Read the model definition and answer for the solid it produces. Units are mm, in the model's axes. A direction names the side the tool comes from. Give positions to 0.01 mm unless a question says otherwise; leave off trailing zeros. Order: outer loops, then holes, each group sorted by start corner. A loop starts at its lowest first (then second) coordinate and runs counter-clockwise, first axis right, second up. Notation, with made-up numbers: M 14,13.25 L 24,13.25 A19 ccw 24,19.25 Z; hole C 20,45.5 d5. An arc over 180 degrees is marked long. Write item = value, one per line. Start each with the question number.
from build123d import *

# Parameters (mm, degrees)
F1_DEPTH = 12.7


with BuildPart() as f1:
    # F0 (on Front) → F1 (new body)
    with BuildSketch(Plane.XZ):
        Polygon((44.074243, -1.927952), (-13.075757, -1.927952), (-13.075757, -8.277952), (15.499243, -8.277952), (44.074243, -8.277952), align=None)
        Polygon((15.499243, -8.277952), (-13.075757, -8.277952), (-41.650757, -8.277952), (-41.650757, -14.627952), (15.499243, -14.627952), align=None)
        Polygon((72.649243, -8.277952), (44.074243, -8.277952), (15.499243, -8.277952), (15.499243, -14.627952), (72.649243, -14.627952), align=None)
    extrude(amount=F1_DEPTH)


solid = f1.part
1) Find section C-C on x = -24. Determine the outline of the cut face in (y, z).
2) For a pull along Y with two mould halves and no side action, classify faces 1 (the face through (15, 0, -10)), 2 (the face through (15, -6, -14.628)), 3 (the face through (15, -12.7, -10)) as pulls with the +Y half, pulls with the -Y half, needs draft (parallel to the pull), parting line crosses it, or undercut.
3) Find the intervals of material crossed by probe 1 along X at (y, z) = (-4.5, -5.5); probe 2 along Z at (x, y) = (49.5, -5.25), in increasing order. Write a range as [from, to].
4) Find section A-A on y = -6.5. Determine the outline of the cut face in (x, z), plus the area to 3 significant figures.
5) For faces 4 (the face through (-27, -6, -8.278)), 5 (the face through (72.649, -6, -11)), 6 (the face through (44.074, -6, -5)), determine the directions among +Z, -Z, +X, -X, +Y, -Y from which every point of the face is accessible in a straight line to the end or side of a thin tool.
6) Each of these flat-tipped pins is pushed along its axis until it touches: P1, Ø6, axis at x = 38.5, z = -5.5, coming from the +Y side; P2, Ø3, axis at y = -6, z = -6, coming from the -X side; P3, Ø4, axis at x = -29, y = -8, coming from the +Z side. Where does it stop, or does it pass through?
7) Find section B-B on z = -4. Determine the outline of the cut face in (x, y).
Numbers:
q1.outline = M -12.7,-14.63 L 0,-14.63 L 0,-8.28 L -12.7,-8.28 Z
q2.face_1 = pulls with the +Y half
q2.face_2 = needs draft
q2.face_3 = pulls with the -Y half
q3.probe_1 = [-13.08, 44.07]
q3.probe_2 = [-14.63, -8.28]
q4.outline = M -41.65,-14.63 L 72.65,-14.63 L 72.65,-8.28 L 44.07,-8.28 L 44.07,-1.93 L -13.08,-1.93 L -13.08,-8.28 L -41.65,-8.28 Z
q4.area = 1,090 mm2
q5.face_4 = +Z, -X, +Y, -Y
q5.face_5 = +Z, -Z, +X, +Y, -Y
q5.face_6 = +Z, +X, +Y, -Y
q6.P1 = 0
q6.P2 = -13.08
q6.P3 = -8.28
q7.outline = M -13.08,-12.7 L 44.07,-12.7 L 44.07,0 L -13.08,0 Z
